For this review, take the finished solid that the model builds, in its own axes (mm). A direction names the side the tool comes from. Coordinates: 2 decimals unless noted, no trailing zeros. Write each loop counter-clockwise with the first axis right and the second up, starting at its lowest first coordinate (ties: lowest second). Pieces come first, ordered by that corner, then holes. Notation, with made-up numbers: M 79.5,58.5 L 110.5,58.5 A5 ccw 110.5,63.5 Z; hole C 18.5,21 d7. An arc over 180 degrees is marked long. One line per question, with ' | ' between items.
from build123d import *

# Parameters (mm, degrees)
SKETCH_1_W          = 58.36
SKETCH_1_H          = 50.07
EXTRUDE_1_DEPTH     = 3
SKETCH_2_W          = 58.36
SKETCH_2_H          = 50.07
SKETCH_2_W_2        = 56.36
SKETCH_2_H_2        = 48.07
EXTRUDE_2_DEPTH     = 7
EXTRUDE_3_DEPTH     = 3
SKETCH_4_W          = 1
SKETCH_4_H          = 1.2
CUT_EXTRUDE_1_DEPTH = 5
EXTRUDE_4_DEPTH     = 15.67
EXTRUDE_5_DEPTH     = 16.67


with BuildPart() as part:
    # 草圖1 → 填料-伸長1 (new body)
    with BuildSketch(Plane.XY):
        with Locations((4.337567568, 6.83036036)):
            Rectangle(SKETCH_1_W, SKETCH_1_H)
    extrude(amount=EXTRUDE_1_DEPTH)

    # 草圖2 → 填料-伸長2 (add)
    with BuildSketch(Plane.XY.offset(3)):
        with Locations((4.337567568, 6.83036036)):
            Rectangle(SKETCH_2_W, SKETCH_2_H)
        with Locations((4.337567568, 6.83036036)):
            Rectangle(SKETCH_2_W_2, SKETCH_2_H_2, mode=Mode.SUBTRACT)
    extrude(amount=EXTRUDE_2_DEPTH)

    # 草圖3 → 填料-伸長3 (add)
    with BuildSketch(Plane.XY.offset(3)):
        Polygon((-23.842432432, 30.86536036), (-23.842432432, 23.86536036), (-16.842432432, 30.86536036), align=None)
        Polygon((32.517567568, -17.20463964), (32.517567568, -10.20463964), (25.517567568, -17.20463964), align=None)
        Polygon((32.517567568, 30.86536036), (32.517567568, 23.86536036), (25.517567568, 30.86536036), align=None)
        Polygon((-23.842432432, -17.20463964), (-23.842432432, -10.20463964), (-16.842432432, -17.20463964), align=None)
    extrude(amount=EXTRUDE_3_DEPTH)

    # 草圖4 → 除料-伸長1 (cut)
    with BuildSketch(Plane.XY.offset(10)):
        with Locations((-24.342432432, -1.60463964)):
            Rectangle(SKETCH_4_W, SKETCH_4_H)
        with Locations((-24.342432432, 16.26536036)):
            Rectangle(SKETCH_4_W, SKETCH_4_H)
        with Locations((33.017567568, -1.60463964)):
            Rectangle(SKETCH_4_W, SKETCH_4_H)
        with Locations((33.017567568, 15.26536036)):
            Rectangle(SKETCH_4_W, SKETCH_4_H)
    extrude(amount=-CUT_EXTRUDE_1_DEPTH, mode=Mode.SUBTRACT)

    # 草圖5 → 填料-伸長4 (add)
    with BuildSketch(Plane.XZ.offset(1.00463964)):
        Polygon((32.517567568, 10), (30.517567568, 7.6), (32.517567568, 7.6), align=None)
    extrude(amount=-EXTRUDE_4_DEPTH)

    # 草圖6 → 填料-伸長5 (add)
    with BuildSketch(Plane.XZ.offset(1.00463964)):
        Polygon((-23.842432432, 10), (-21.842432432, 7.6), (-23.842432432, 7.6), align=None)
    extrude(amount=-EXTRUDE_5_DEPTH)


solid = part.part
1. Machinability: for faces 1 (the flat face through (4, 7, 0)), 2 (the flat face through (-24, -1.005, 8)), 3 (the flat face through (32.518, 6, 6)), 4 (the flat face through (33, 14.665, 8)), 5 (the flat face through (29.067, 27.316, 4.479)), which of the approach directions +Z, -Z, +X, -X, +Y, -Y give a long, thin tool a straight path to every point of the face, cutting with its end or side? Answer none if there is none.
Computed values:
face 1: -Z, +X, -X, +Y, -Y | face 2: +Z, +X, -X | face 3: none | face 4: +Z, +X | face 5: +Z
2. Take a section at A-A on z = 4. State the section outline as (x, y) points.
Computed values:
outline: M -24.84,-18.2 L 33.52,-18.2 L 33.52,31.87 L -24.84,31.87 Z; hole M -23.84,-10.2 L -16.84,-17.2 L 25.52,-17.2 L 32.52,-10.2 L 32.52,23.87 L 25.52,30.87 L -16.84,30.87 L -23.84,23.87 Z
3. Take a section at D-D on y = 8. State the section outline as (x, z) points.
Computed values:
outline: M -24.84,0 L 33.52,0 L 33.52,10 L 32.52,10 L 30.52,7.6 L 32.52,7.6 L 32.52,3 L -23.84,3 L -23.84,7.6 L -21.84,7.6 L -23.84,10 L -24.84,10 Z
4. Take a section at B-B on x = 11. State the section outline as (y, z) points, plus the area to 3 significant figures.
Computed values:
outline: M -18.2,0 L 31.87,0 L 31.87,10 L 30.87,10 L 30.87,3 L -17.2,3 L -17.2,10 L -18.2,10 Z | area: 164 mm2
5. Draft analysis for pull direction X (two halves, no side actions). For faces 6 (the flat face through (-24.842, 6, 5)), 7 (the flat face through (31, -15, 6)), 8 (the flat face through (33, -1.005, 8)), 9 (the flat face through (33.518, 6, 5)), state which applies: pulls with the +X half, pulls with the -X half, needs draft (parallel to the pull), parting line crosses it, or undercut.
Computed values:
face 6: pulls with the -X half | face 7: undercut | face 8: needs draft | face 9: pulls with the +X half
6. Take a section at C-C on z = 8.5. State the section outline as (x, y) points, plus the area to 3 significant figures.
Computed values:
outline: M -24.84,-18.2 L 33.52,-18.2 L 33.52,-2.2 L 32.52,-2.2 L 32.52,-17.2 L -23.84,-17.2 L -23.84,-2.2 L -24.84,-2.2 Z; M -24.84,-1 L -22.59,-1 L -22.59,15.67 L -24.84,15.67 Z; M -24.84,16.87 L -23.84,16.87 L -23.84,30.87 L 32.52,30.87 L 32.52,15.87 L 33.52,15.87 L 33.52,31.87 L -24.84,31.87 Z; M 31.27,-1 L 33.52,-1 L 33.52,14.67 L 31.27,14.67 Z | area: 248 mm2
7. Clearance check with flat-ended pins moving along their axes: P1, Ø0.5, axis at x = -24.5, y = -1.5, coming from the +Z side; P2, Ø1.5, axis at x = 27, y = 20, coming from the +Z side; P3, Ø2, axis at x = 29.5, y = 28.5, coming from the +Z side. State where each tip first meets the part, or that it passes through.
Computed values:
P1: stops at z = 5 | P2: stops at z = 3 | P3: stops at z = 6
8. For line 1 along Y through (x, z) = (25.5, 4.5); line 2 along X through (y, z) = (-4, 4); line 3 along Z through (x, y) = (-5, -14), list the stretches that pass through material, from the lowest coordinate up.
Computed values:
line 1: y = -18.2 to -17.2, 30.87 to 31.87 | line 2: x = -24.84 to -23.84, 32.52 to 33.52 | line 3: z = 0 to 3
